Design review of the part built by this model. Coordinates are the model's own, in mm. A direction names the side the tool comes from. Give positions to 0.01 mm unless a question says otherwise; leave off trailing zeros. Loops run counter-clockwise (first coordinate to the right, second up) from the corner with the lowest first, then second, coordinate; pieces in that order, holes last. Notation, with made-up numbers: (89.25, -35.5) -> (101.25, -35.5) arc R4 ccw to (101.25, -29.5) -> close; hole circle Ø8 at (3.5, 0). An arc over 180 degrees is marked (long way). Answer in a Markdown table with one row per item. Add a question column.
(1) For line 1 (X direction, y = 4.75, z = -11.5); line 2 (X direction, y = -7, z = 13.5); line 3 (Z direction, x = 83, y = 9), list the stretches that pass through material, from the lowest coordinate up.
(2) For pin 1 (3 mm diameter, centred on x = 28, y = -1.5, fed in from -Z); pin 2 (1.9 mm diameter, centred on y = -2.5, z = 30.5, fed in from +X); pin 3 (3 mm diameter, centred on x = 47, y = 9.5, fed in from -Z), all flat-tipped, find the tip position at first contact; note any pin that passes through.
(3) Consider section A-A on y = -4. Write out the cut boundary in (x, z).
(4) For faces 1 (the cylindrical face through (-1.528, 11.251, 30.914)), 2 (the cylindrical face through (-1.528, 11.251, -30.891)), 3 (the cylindrical face through (-1.528, -11.251, 30.914)), 4 (the cylindrical face through (-1.528, -11.251, -30.891)), list the 3-axis set-ups (+Z, -Z, +X, -X, +Y, -Y) from which the entire face can be reached by the end or side of a thin tool; tool diameter is ignored.
from build123d import *

# Parameters (mm, degrees)
F1_DEPTH = 12.7
F2_R     = 5.08
F3_R     = 5.08


with BuildPart() as f1:
    # F0 (on Front) → F1 (new body, symmetric)
    with BuildSketch(Plane.XZ):
        Polygon((0, -31.75), (0, -25.4), (0, 25.4), (0, 31.75), (-19.05, 31.75), (-19.05, -31.75), align=None)
        Polygon((0, 25.4), (0, -25.4), (108.871248, -15.875), (108.871248, 15.875), align=None)
    extrude(amount=F1_DEPTH, both=True)

    # F2
    f2_edges = [f1.edges().sort_by_distance(p)[0] for p in [
        (0, 0, 25.4),
        (0, 0, -25.4),
    ]]
    fillet(f2_edges, radius=F2_R)

    # F3
    f3_edges = [f1.edges().sort_by_distance(p)[0] for p in [
        (56.754249, 12.7, 20.434647),
        (108.871248, 0, 15.875),
        (56.754249, -12.7, 20.434647),
        (108.871248, -12.7, 0),
        (108.871248, 12.7, 0),
        (56.754249, -12.7, -20.434647),
        (56.754249, 12.7, -20.434647),
        (108.871248, 0, -15.875),
    ]]
    fillet(f3_edges, radius=F3_R)


solid = f1.part
Values follow:
| question | item | result |
|---|---|---|
| 1 | line 1 | -19.05 to 108.86 |
| 1 | line 2 | -19.05 to 108.33 |
| 1 | line 3 | -17.95 to 17.95 |
| 2 | pin 1 | z = -23.08 |
| 2 | pin 2 | x = 0.03 |
| 2 | pin 3 | z = -21.32 |
| 3 | outline | (-19.05, -31.75) -> (0, -31.75) -> (0, -30.05) arc R5.08 cw to (4.64, -24.99) -> (104.23, -16.28) arc R5.08 ccw to (108.87, -11.22) -> (108.87, 11.22) arc R5.08 ccw to (104.23, 16.28) -> (4.64, 24.99) arc R5.08 cw to (0, 30.05) -> (0, 31.75) -> (-19.05, 31.75) -> close |
| 4 | face 1 | +Z, +X, +Y |
| 4 | face 2 | -Z, +X, +Y |
| 4 | face 3 | +Z, +X, -Y |
| 4 | face 4 | -Z, +X, -Y |
